Could you check a few things on this model? Use its own coordinates, in mm. A direction names the side the tool comes from. Give positions to 0.01 mm unless a question says otherwise; leave off trailing zeros. Order: outer loops, then holes, each group sorted by start corner. A loop starts at its lowest first (then second) coordinate and runs counter-clockwise, first axis right, second up. Notation, with made-up numbers: (-16, 73.25) - (14, 73.25) arc R33 ccw to (14, 111.25) - close; hole circle Ø1 at (49, 65). An arc over 180 degrees is marked (long way). One line per question, with ' | ' between items. Start each with the question number.
1. I need wall thicknesses on probe 1 along X at (y, z) = (-1, 11.25); probe 2 along Z at (x, y) = (-4.5, 38); probe 3 along Y at (x, z) = (7.5, -18). Which ranges of each line are inside material? Lowest first, please. Write a range as from..to.
2. Imagine slicing it at B-B (z = 11.25). Please give me the cut outline in (x, y), and give its area (3 significant figures).
3. For P1, Ø2.5, axis at x = -7.75, y = 32.92, coming from the +Z side; P2, Ø2, axis at x = -0.5, z = 3.5, coming from the +Y side; P3, Ø10, axis at x = -7, y = 33.5, coming from the -Z side, each with a flat end and sliding along its axis, tell me the tip position at first contact or that it passes through.
4. Imagine slicing it at C-C (x = 8). Please give me the cut outline in (y, z), and give its area (3 significant figures).
5. Imagine slicing it at D-D (x = 15.5). Please give me the cut outline in (y, z).
6. If we mould it in two halves opening along Z, with no side actions, what happens to faces 1 (the flat face through (9, 14, 20.25)), 2 (the cylindrical face through (16.68, 20.58, 19.24)), 3 (the cylindrical face through (15.941, -0.986, -14.226)), 4 (the cylindrical face through (15.941, -0.986, 9.774))? For each: released by +Z, released by -Z, zero draft, split by the parting line, or undercut.
7. Imagine slicing it at A-A (y = 16.5). Please give me the cut outline in (x, z), and give its area (3 significant figures).
8. Which directions (+Z, -Z, +X, -X, +Y, -Y) give clear straight access to the entire face, cutting with the end or side of a thin tool? Please do faces 5 (the flat face through (0, 0, -1)), 6 (the flat face through (20, -1, 5)), 7 (the flat face through (6.5, 19, 19)).
```python
from build123d import *

# Parameters (mm, degrees)
EXTRUDE_1_DEPTH             = 40.5
SKETCH_2_W                  = 38.5
SKETCH_2_H                  = 19.5
CUT_EXTRUDE_1_DEPTH         = 60.752092014
CUT_EXTRUDE_2_DEPTH         = 2
HOLE_WIZARD_3_5_3_5_1_D     = 3.5
HOLE_WIZARD_3_5_3_5_1_DEPTH = 2
HOLE_WIZARD_3_2_3_2_1_D     = 3.2
HOLE_WIZARD_3_2_3_2_1_DEPTH = 40.5
SKETCH_12_R                 = 1.6
CUT_EXTRUDE_3_DEPTH         = 38.5


with BuildPart() as part:
    # 草图1 → 凸台-拉伸1 (new body)
    with BuildSketch(Plane.XY.offset(20.25)):
        with BuildLine():
            Line((20, -2), (20, 19.5))
            ThreePointArc((20, 19.5), (0, 39.5), (-20, 19.5))
            Line((-20, 19.5), (-20, -2))
            Line((-20, -2), (20, -2))
        make_face()
    extrude(amount=-EXTRUDE_1_DEPTH)

    # 草图2 → 切除-拉伸1 (cut, through all)
    with BuildSketch(Plane(origin=(20, 0, 0), x_dir=(0, 0, -1), z_dir=(1, 0, 0))):
        with Locations((1, 9.75)):
            Rectangle(SKETCH_2_W, SKETCH_2_H)
    extrude(amount=-CUT_EXTRUDE_1_DEPTH, mode=Mode.SUBTRACT)

    # 草图3 → 切除-拉伸2 (cut)
    with BuildSketch(Plane.XY.offset(20.25)):
        with BuildLine():
            Line((-6.5, 26.5), (-6.5, 12.5))
            ThreePointArc((-6.5, 12.5), (0, 6), (6.5, 12.5))
            Line((6.5, 12.5), (6.5, 26.5))
            ThreePointArc((6.5, 26.5), (0, 33), (-6.5, 26.5))
        make_face()
    extrude(amount=-CUT_EXTRUDE_2_DEPTH, mode=Mode.SUBTRACT)

    # Ø3.5 (3.5) 直径孔1
    with Locations(Plane(origin=(0, -2, 0), x_dir=(-1, 0, 0), z_dir=(0, -1, 0))):
        with Locations((15, -11.25), (15, 12.75), (-15, 12.75), (-15, -11.25)):
            Hole(HOLE_WIZARD_3_5_3_5_1_D / 2, depth=HOLE_WIZARD_3_5_3_5_1_DEPTH)

    # Ø3.2 (3.2) 直径孔1
    with Locations(Plane.XY.offset(20.25)):
        with Locations((-7.75, 32.923393759), (-7.75, 6.076606241), (15.5, 19.5), (7.75, 6.076606241), (-15.5, 19.5), (7.75, 32.923393759)):
            Hole(HOLE_WIZARD_3_2_3_2_1_D / 2, depth=HOLE_WIZARD_3_2_3_2_1_DEPTH)

    # 草图12 → 切除-拉伸3 (cut)
    with BuildSketch(Plane(origin=(0, 0, -20.25), x_dir=(-1, 0, 0), z_dir=(0, 0, -1))):
        with BuildLine():
            Line((-20, 19.5), (-17.1, 19.5))
            ThreePointArc((-17.1, 19.5), (-15.5, 21.1), (-13.9, 19.5))
            Line((-13.9, 19.5), (13.9, 19.5))
            ThreePointArc((13.9, 19.5), (15.5, 21.1), (17.1, 19.5))
            Line((17.1, 19.5), (20, 19.5))
            ThreePointArc((20, 19.5), (0, 39.5), (-20, 19.5))
        make_face()
        with Locations(Location((-7.75, 32.923393759, 0), (0, 0, 180))):
            Circle(SKETCH_12_R, mode=Mode.SUBTRACT)
        with Locations(Location((7.75, 32.923393759, 0), (0, 0, 180))):
            Circle(SKETCH_12_R, mode=Mode.SUBTRACT)
    extrude(amount=-CUT_EXTRUDE_3_DEPTH, mode=Mode.SUBTRACT)


solid = part.part
```
Results found:
1) probe 1: x = -20..-16.75, -13.25..13.25, 16.75..20 | probe 2: z = 18.25..20.25 | probe 3: y = -2..0
2) outline: (-20, -2) - (-16.75, -2) - (-16.75, 0) - (-20, 0) - close; (-13.25, -2) - (13.25, -2) - (13.25, 0) - (-13.25, 0) - close; (16.75, -2) - (20, -2) - (20, 0) - (16.75, 0) - close | area: 66.0 mm2
3) P1: passes through | P2: stops at y = 0 | P3: stops at z = 18.25
4) outline: (-2, -20.25) - (0, -20.25) - (0, 18.25) - (4.5, 18.25) - (4.5, 20.25) - (-2, 20.25) - close; (7.66, 18.25) - (31.34, 18.25) - (31.34, 20.25) - (7.66, 20.25) - close; (34.5, 18.25) - (37.83, 18.25) - (37.83, 20.25) - (34.5, 20.25) - close | area: 144 mm2
5) outline: (-2, -20.25) - (0, -20.25) - (0, -14.43) - (-2, -14.43) - close; (-2, -11.07) - (0, -11.07) - (0, 9.57) - (-2, 9.57) - close; (-2, 12.93) - (0, 12.93) - (0, 18.25) - (17.9, 18.25) - (17.9, 20.25) - (-2, 20.25) - close; (21.1, 18.25) - (32.14, 18.25) - (32.14, 20.25) - (21.1, 20.25) - close
6) face 1: released by +Z | face 2: zero draft | face 3: undercut | face 4: undercut
7) outline: (-20, 18.25) - (-6.5, 18.25) - (-6.5, 20.25) - (-20, 20.25) - close; (6.5, 18.25) - (20, 18.25) - (20, 20.25) - (6.5, 20.25) - close | area: 54.0 mm2
8) face 5: -Z, +X, -X, +Y | face 6: +Z, -Z, +X, +Y, -Y | face 7: +Z, -Z
